Can you work these out from the model? Positions are in its coordinate system, mm. A direction names the side the tool comes from. Give positions to 0.01 mm unless a question says otherwise; leave off trailing zeros. Order: outer loops, then holes, each group sorted by start corner. A loop starts at its lowest first (then second) coordinate and runs counter-clockwise, first axis right, second up.
Item 1: Which directions (+Z, -Z, +X, -X, +Y, -Y) give clear straight access to the entire face, cutting with the end or side of a thin tool? Please do faces 4 (the cylindrical face through (19.65, -1.01, 0.57)), 5 (the cylindrical face through (16.12, 2.74, 1.93)), 6 (the cylindrical face through (3.35, -1.01, 3.43)), 7 (the cylindrical face through (19.65, -1.01, 3.43)).
Item 2: I want a section at D-D, the plane y = 2.25. Write out the boundary of the cut face in (x, z) (3 decimals).
Item 3: If we mould it in two halves opening along X, with no side actions, what happens to faces 1 (the cylindrical face through (3.35, -1.01, 0.57)), 2 (the cylindrical face through (1.21, 0.49, 2.69)), 3 (the flat face through (11, 0, 4))? For each: +X half, -X half, draft (parallel to the pull), parting line (faces both ways), or undercut.
Item 4: I want a section at A-A, the plane x = 21.25. Write out the boundary of the cut face in (y, z), then the cut area to 3 significant figures.
Item 5: I'm going to push flat-ended pins straight in: pin 1 Ø2 at (x, z) = (3, 1.5) entering from +Y; pin 2 Ø1 at (y, z) = (-1, 1.5) entering from -X; pin 3 Ø2 at (x, y) = (16, 2.5) entering from +Z. Where does each tip first touch, or does it pass through?
Item 6: I want a section at C-C, the plane x = 4. Write out the boundary of the cut face in (y, z).
Item 7: If I drill on line 1 along X through (y, z) = (0.65, 2); line 2 along Y through (x, z) = (14.5, 2.5); line 3 along Y through (x, z) = (3.5, 0.4), over which ranges is the centre line in solid material (lowest first)?
Item 8: I want a section at B-B, the plane z = 0.9. Write out the boundary of the cut face in (x, y), then the cut area to 3 significant figures.
```python
from build123d import *

# Parameters (mm, degrees)
SKETCH1_W           = 23
SKETCH1_H           = 4
SKETCH1_R           = 0.75
BOSS_EXTRUDE1_DEPTH = 1
SKETCH2_W           = 17.5
SKETCH2_H           = 4
BOSS_EXTRUDE2_DEPTH = 1
SKETCH3_W           = 17.5
SKETCH3_H           = 4
BOSS_EXTRUDE3_DEPTH = 2
SKETCH4_R           = 0.5
BOSS_EXTRUDE4_DEPTH = 1.5
FILLET1_R           = 2
FILLET2_R           = 2


with BuildPart() as part:
    # Sketch1 → Boss-Extrude1 (new body)
    with BuildSketch(Plane(origin=(0, 0, 0), x_dir=(1, 0, 0), z_dir=(0, 1, 0))):
        with Locations((11.5, -2)):
            Rectangle(SKETCH1_W, SKETCH1_H)
        with Locations(Location((1.5, -2, 0), (0, 0, 270))):
            Circle(SKETCH1_R, mode=Mode.SUBTRACT)
        with Locations(Location((21.5, -2, 0), (0, 0, 270))):
            Circle(SKETCH1_R, mode=Mode.SUBTRACT)
    extrude(amount=BOSS_EXTRUDE1_DEPTH)

    # Sketch2 → Boss-Extrude2 (add)
    with BuildSketch(Plane(origin=(0, 1, 0), x_dir=(1, 0, 0), z_dir=(0, 1, 0))):
        with Locations((11.5, -2)):
            Rectangle(SKETCH2_W, SKETCH2_H)
    extrude(amount=BOSS_EXTRUDE2_DEPTH)

    # Sketch3 → Boss-Extrude3 (add)
    with BuildSketch(Plane(origin=(0, 0, 0), x_dir=(-1, 0, 0), z_dir=(0, -1, 0))):
        with Locations((-11.5, -2)):
            Rectangle(SKETCH3_W, SKETCH3_H)
    extrude(amount=BOSS_EXTRUDE3_DEPTH)

    # Sketch4 → Boss-Extrude4 (add)
    with BuildSketch(Plane(origin=(0, 2, 0), x_dir=(1, 0, 0), z_dir=(0, 1, 0))):
        with Locations(Location((7.375, -2, 0), (0, 0, 270))):
            Circle(SKETCH4_R)
        with Locations(Location((10.125, -2, 0), (0, 0, 270))):
            Circle(SKETCH4_R)
        with Locations(Location((12.875, -2, 0), (0, 0, 270))):
            Circle(SKETCH4_R)
        with Locations(Location((15.625, -2, 0), (0, 0, 270))):
            Circle(SKETCH4_R)
    extrude(amount=BOSS_EXTRUDE4_DEPTH)

    # Fillet1
    fillet1_edges = [part.edges().sort_by_distance(p)[0] for p in [
        (20.25, -1, 4),
        (20.25, -1, 0),
        (20.25, 1.5, 0),
        (20.25, 1.5, 4),
        (2.75, 1.5, 4),
        (2.75, 1.5, 0),
        (2.75, -1, 0),
        (2.75, -1, 4),
    ]]
    fillet(fillet1_edges, radius=FILLET1_R - 0.0001)  # a hair under: the kernel refuses the full size

    # Fillet2
    fillet2_edges = [part.edges().sort_by_distance(p)[0] for p in [
        (0, 0.5, 4),
        (0, 0.5, 0),
        (23, 0.5, 0),
        (23, 0.5, 4),
    ]]
    fillet(fillet2_edges, radius=FILLET2_R - 0.0001)  # a hair under: the kernel refuses the full size


solid = part.part
```
Results list:
1. face 4: -Z, +X, -Y
1. face 5: +Y
1. face 6: +Z, -X, -Y
1. face 7: +Z, +X, -Y
2. outline: circle Ø1 at (7.375, 2); circle Ø1 at (10.125, 2); circle Ø1 at (12.875, 2); circle Ø1 at (15.625, 2)
3. face 1: -X half
3. face 2: undercut
3. face 3: draft
4. outline: (0, 0.02) - (1, 0.02) - (1, 1.29) - (0, 1.29) - close; (0, 2.71) - (1, 2.71) - (1, 3.98) - (0, 3.98) - close
4. area: 2.55 mm2
5. pin 1: stops at y = 2
5. pin 2: stops at x = 2.75
5. pin 3: stops at z = 4
6. outline: (-2, 0.15) - (0, 0.15) - (0, 0) - (1, 0) - (1, 0.15) - (2, 0.15) - (2, 3.85) - (1, 3.85) - (1, 4) - (0, 4) - (0, 3.85) - (-2, 3.85) - close
7. line 1: x = 0 to 0.75, 2.25 to 20.75, 22.25 to 23
7. line 2: y = -2 to 2
7. line 3: y = 0 to 1
8. outline: (0.33, 0) - (3.08, 0) - (3.08, -2) - (19.92, -2) - (19.92, 0) - (22.67, 0) - (22.67, 1) - (19.92, 1) - (19.92, 2) - (3.08, 2) - (3.08, 1) - (0.33, 1) - close
8. area: 72.9 mm2
